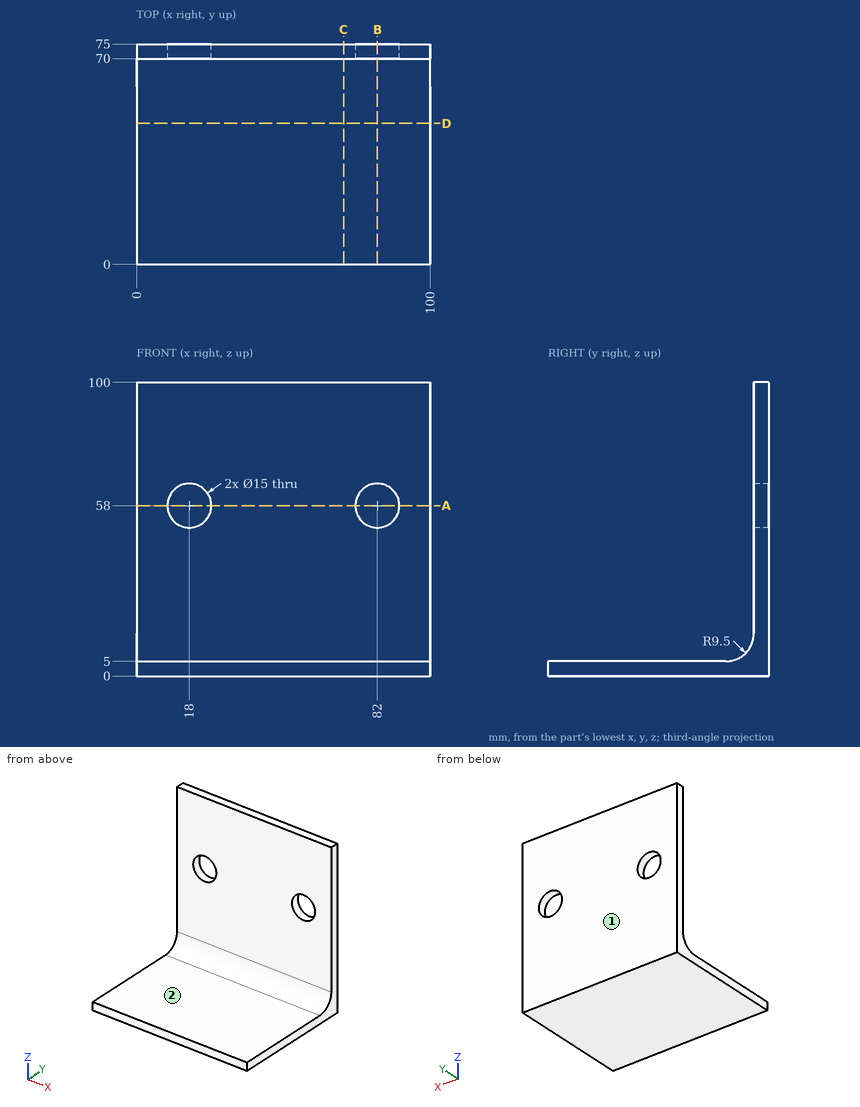
Study the drawing (mm; zero at the part's minimum x, y, z) and answer. A direction names the side the tool comes from. Give positions to 0.01 mm unless a question says otherwise; leave off trailing zeros. Order: outer loops, then holes, each group sorted by start corner. A loop starts at its lowest first (then second) coordinate and runs counter-clockwise, first axis right, second up.
1. Section C-C, the plane x = 70.5 is taken. Determine the outline of the cut face in (y, z).
Result sheet:
outline: (0, 0) - (75, 0) - (75, 100) - (70, 100) - (70, 14.5) arc R9.5 cw to (60.5, 5) - (0, 5) - close
2. Straight lines are drawn through the part: L1, parallel to Z at x = 82, y = 72.25; L2, parallel to Y at x = 19.5, z = 44; L3, parallel to Z at x = 14, y = 12. For each, find the intervals that lie inside material, in ascending order.
Result sheet:
L1: z = 0 to 50.5, 65.5 to 100
L2: y = 70 to 75
L3: z = 0 to 5
3. Section A-A, the plane z = 58 is taken. Determine the outline of the cut face in (x, y), and give its area (3 significant figures).
Result sheet:
outline: (0, 70) - (10.5, 70) - (10.5, 75) - (0, 75) - close; (25.5, 70) - (74.5, 70) - (74.5, 75) - (25.5, 75) - close; (89.5, 70) - (100, 70) - (100, 75) - (89.5, 75) - close
area: 350 mm2
4. Section D-D, the plane y = 48 is taken. Determine the outline of the cut face in (x, z), and give its area (3 significant figures).
Result sheet:
outline: (0, 0) - (100, 0) - (100, 5) - (0, 5) - close
area: 500 mm2
5. Section B-B, the plane x = 82 is taken. Determine the outline of the cut face in (y, z), and give its area (3 significant figures).
Result sheet:
outline: (0, 0) - (75, 0) - (75, 50.5) - (70, 50.5) - (70, 14.5) arc R9.5 cw to (60.5, 5) - (0, 5) - close; (70, 65.5) - (75, 65.5) - (75, 100) - (70, 100) - close
area: 794 mm2
6. For the marked faces 1 and 2, determine the directions among +Z, -Z, +X, -X, +Y, -Y from which every point of the face is accessible in a straight line to the end or side of a thin tool.
Result sheet:
face 1: +Z, -Z, +X, -X, +Y
face 2: +Z, +X, -X, -Y
7. Each of these flat-tipped pins is pushed along its axis until it touches: P1, Ø10, axis at x = 72, y = 36, coming from the +Z side; P2, Ø17, axis at x = 18, z = 58, coming from the -Y side; P3, Ø9, axis at x = 82, z = 58, coming from the -Y side. Where does it stop, or does it pass through?
Result sheet:
P1: stops at z = 5
P2: stops at y = 70
P3: passes through
